Geometry: see drawing. Coordinates: mm, zero at the bounding-box minimum. A direction names the side the tool comes from. Give positions to 0.01 mm unless a question says otherwise; leave off trailing zeros. Write each loop counter-clockwise with the first axis right and the second up, starting at its lowest first coordinate (ties: lowest second). Pieces come first, ordered by that corner, then holes. Notation, with made-up numbers: M -30.5,23 L 15.5,23 A24 cw 15.5,36 Z; hole C 19,-4.75 d4. An arc over 180 degrees is marked long. Use CSV: the item, a comma, the result in double quotes. Start each with the question number.
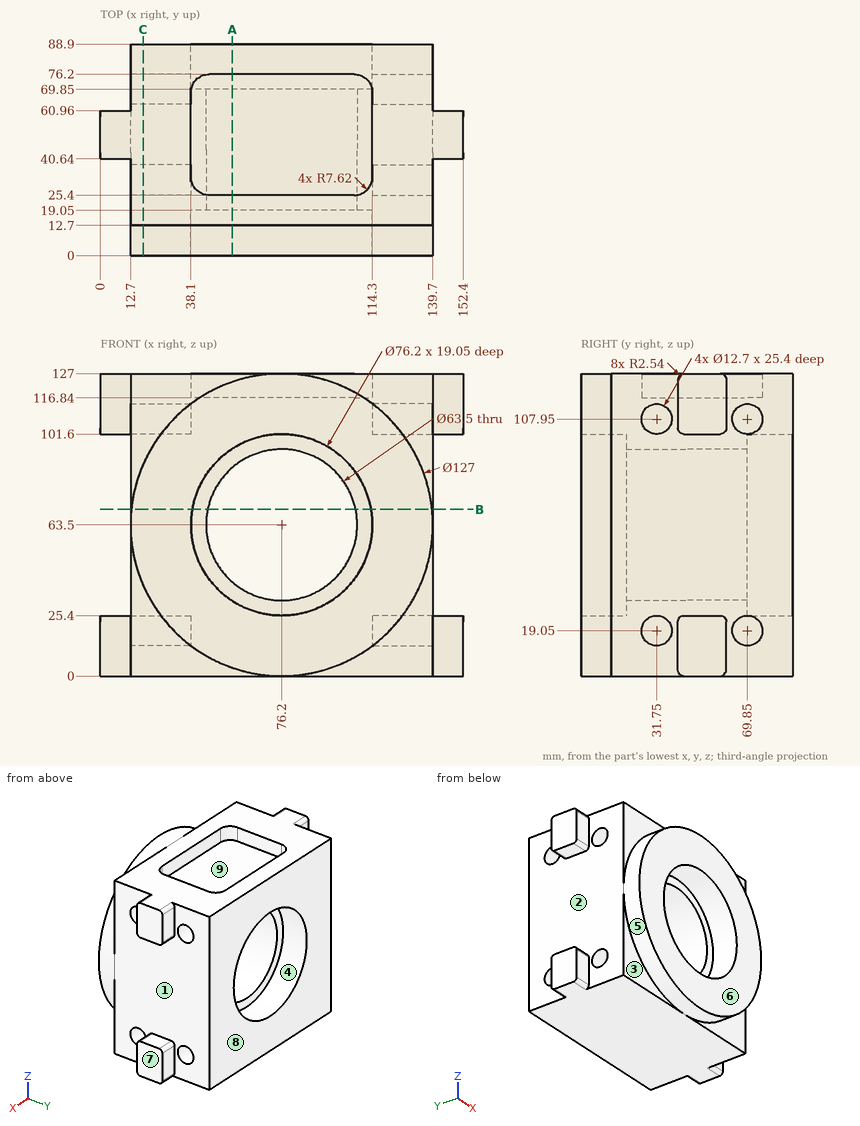
1. Access query for the marked faces 1, 2, 3, 4 and 5. Directions: +Z, -Z, +X, -X, +Y, -Y. A direction counts if a zero-diameter tool reaches every point of the face in a straight line with its end or side. Return the directions, or none.
2. Section C-C on x = 18. Return loops of the section in (y, z), then the cut area to 3 significant figures.
3. First-contact query: pin 1 (14 mm diameter, centred on x = 146, z = 114, fed in from -Y); pin 2 (6 mm diameter, centred on y = 44.5, z = 76.5, fed in from +X); pin 3 (16.5 mm diameter, centred on y = 69.85, z = 19.05, fed in from -X); pin 4 (3 mm diameter, centred on y = 49.5, z = 122, fed in from -X). Flat tips, straight axial feed; report the tip coordinate or a pass-through.
4. Line query: probe 1 along Y at (x, z) = (26, 19); probe 2 along X at (y, z) = (55.5, 64); probe 3 along Z at (x, y) = (76.2, 15). Output: solid intervals per line, ascending.
5. Section B-B on z = 70. Return loops of the section in (x, y), then the cut area to 3 significant figures.
6. Section A-A on x = 55.5. Return loops of the section in (y, z), then the cut area to 3 significant figures.
7. Pull-direction query (Y, two-part tool) for the marked faces 6, 7, 8 and 9; classes: released by +Y, released by -Y, zero draft, split by the parting line, or undercut.
Resolved:
1,face 1,"+X"
1,face 2,"-X"
1,face 3,"-Z, -X, -Y"
1,face 4,"+Y"
1,face 5,"-Y"
2,outline,"M 0,38.1 L 12.7,38.1 L 12.7,0 L 88.9,0 L 88.9,127 L 12.7,127 L 12.7,88.9 L 0,88.9 Z; hole C 31.75,19.05 d12.7; hole C 31.75,107.95 d12.7; hole C 69.85,19.05 d12.7; hole C 69.85,107.95 d12.7"
2,area,"9,820 mm2"
3,pin 1,"stops at y = 12.7"
3,pin 2,"stops at x = 139.7"
3,pin 3,"stops at x = 12.7"
3,pin 4,"stops at x = 0"
4,probe 1,"y = 12.7 to 25.4, 38.1 to 63.5, 76.2 to 88.9"
4,probe 2,"x = 12.7 to 44.45, 107.95 to 139.7"
4,probe 3,"z = 0 to 25.4, 101.6 to 127"
5,outline,"M 12.7,12.7 L 13.03,12.7 L 13.03,0 L 38.66,0 L 38.66,19.05 L 45.12,19.05 L 45.12,69.85 L 38.66,69.85 L 38.66,88.9 L 12.7,88.9 Z; M 107.28,19.05 L 113.74,19.05 L 113.74,0 L 139.37,0 L 139.37,12.7 L 139.7,12.7 L 139.7,88.9 L 113.74,88.9 L 113.74,69.85 L 107.28,69.85 Z"
5,area,"5,260 mm2"
6,outline,"M 0,3.47 L 12.7,3.47 L 12.7,0 L 88.9,0 L 88.9,31.51 L 69.85,31.51 L 69.85,39.43 L 19.05,39.43 L 19.05,31.51 L 0,31.51 Z; M 0,95.49 L 19.05,95.49 L 19.05,87.57 L 69.85,87.57 L 69.85,95.49 L 88.9,95.49 L 88.9,127 L 76.2,127 L 76.2,116.84 L 25.4,116.84 L 25.4,127 L 12.7,127 L 12.7,123.53 L 0,123.53 Z"
6,area,"5,800 mm2"
7,face 6,"released by -Y"
7,face 7,"zero draft"
7,face 8,"released by +Y"
7,face 9,"undercut"
